Here's how the part is built. I have some questions about the finished solid (model axes, mm). A direction names the side the tool comes from. Round coordinates to 2 decimals unless told otherwise and drop trailing zeros. Loops run counter-clockwise (first coordinate to the right, second up) from the corner with the lowest first, then second, coordinate; pieces in that order, holes last. Notation, with made-up numbers: M -25.5,23 L 21.5,23 A16 ccw 21.5,39 Z; hole C -23,22 d6. An arc over 180 degrees is marked long. Answer as CSV lines item,"result".
```python
from build123d import *

# Parameters (mm, degrees)
F0_R     = 4.699
F1_DEPTH = 8.89
F2_R     = 2.5
F3_DEPTH = 25.4
F4_R     = 3.556
F5_DEPTH = 6.35


# Not quite as in the source:
# - a feature names something its author has since deleted; it is built from what else it names


with BuildPart() as f1:
    # F0 (on Top) → F1 (new body)
    with BuildSketch(Plane.XY):
        Circle(F0_R)
    extrude(amount=F1_DEPTH)

    # F2 (on face) → F3 (join)
    with BuildSketch(Plane.XY.offset(8.89)):
        Circle(F2_R)
    extrude(amount=F3_DEPTH)

    # F4 (on face) → F5 (cut)
    with BuildSketch(Plane(origin=(0, 0, 0), x_dir=(1, 0, 0), z_dir=(0, 0, -1))):
        Circle(F4_R)
    extrude(amount=-F5_DEPTH, mode=Mode.SUBTRACT)


solid = f1.part
```
1. I want a section at C-C, the plane z = 7. Please give me the cut outline in (x, y), and give its area (3 significant figures).
Evaluation:
outline,"C 0,0 d9.4"
area,"69.4 mm²"
2. I want a section at D-D, the plane y = 3.25. Please give me the cut outline in (x, z), and give its area (3 significant figures).
Evaluation:
outline,"M -3.39,0 L -1.44,0 L -1.44,6.35 L 1.44,6.35 L 1.44,0 L 3.39,0 L 3.39,8.89 L -3.39,8.89 Z"
area,"42.0 mm²"
3. I want a section at A-A, the plane y = 0. Please give me the cut outline in (x, z).
Evaluation:
outline,"M -4.7,0 L -3.56,0 L -3.56,6.35 L 3.56,6.35 L 3.56,0 L 4.7,0 L 4.7,8.89 L 2.5,8.89 L 2.5,34.29 L -2.5,34.29 L -2.5,8.89 L -4.7,8.89 Z"
4. For P1, Ø2, axis at x = 1.5, y = 0.5, coming from the -Z side; P2, Ø3, axis at x = 0, z = 16.5, coming from the -Y side, each with a flat end and sliding along its axis, tell me the tip position at first contact or that it passes through.
Evaluation:
P1,"stops at z = 6.35"
P2,"stops at y = -2.5"
5. If I drill on line 1 (Z direction, x = -3.75, y = 0.75); line 2 (Z direction, x = -2.5, y = 0.75); line 3 (Y direction, x = 2, z = 3.5), over which ranges is the centre line in solid material (lowest first)? Write a range as [from, to].
Evaluation:
line 1,"z = [0, 8.89]"
line 2,"z = [6.35, 8.89]"
line 3,"y = [-4.25, -2.94], [2.94, 4.25]"
6. Which directions (+Z, -Z, +X, -X, +Y, -Y) give clear straight access to the entire face, cutting with the end or side of a thin tool? Please do faces 1 (the flat face through (0, 0, 6.35)), 2 (the flat face through (-1, 4, 0)), 3 (the cylindrical face through (-0.54, -2.44, 21.41)).
Evaluation:
face 1,"-Z"
face 2,"-Z, +X, -X, +Y, -Y"
face 3,"+Z"
7. We'd pull the mould along X, two halves only. Please class faces 4 (the cylindrical face through (-0.77, 3.47, 3.13)), 5 (the flat face through (2, -2, 8.89)), 6 (the cylindrical face through (-0.61, 4.66, 4.38)): pulls with the +X half, pulls with the -X half, needs draft (parallel to the pull), parting line crosses it, or undercut.
Evaluation:
face 4,"undercut"
face 5,"needs draft"
face 6,"parting line crosses it"
